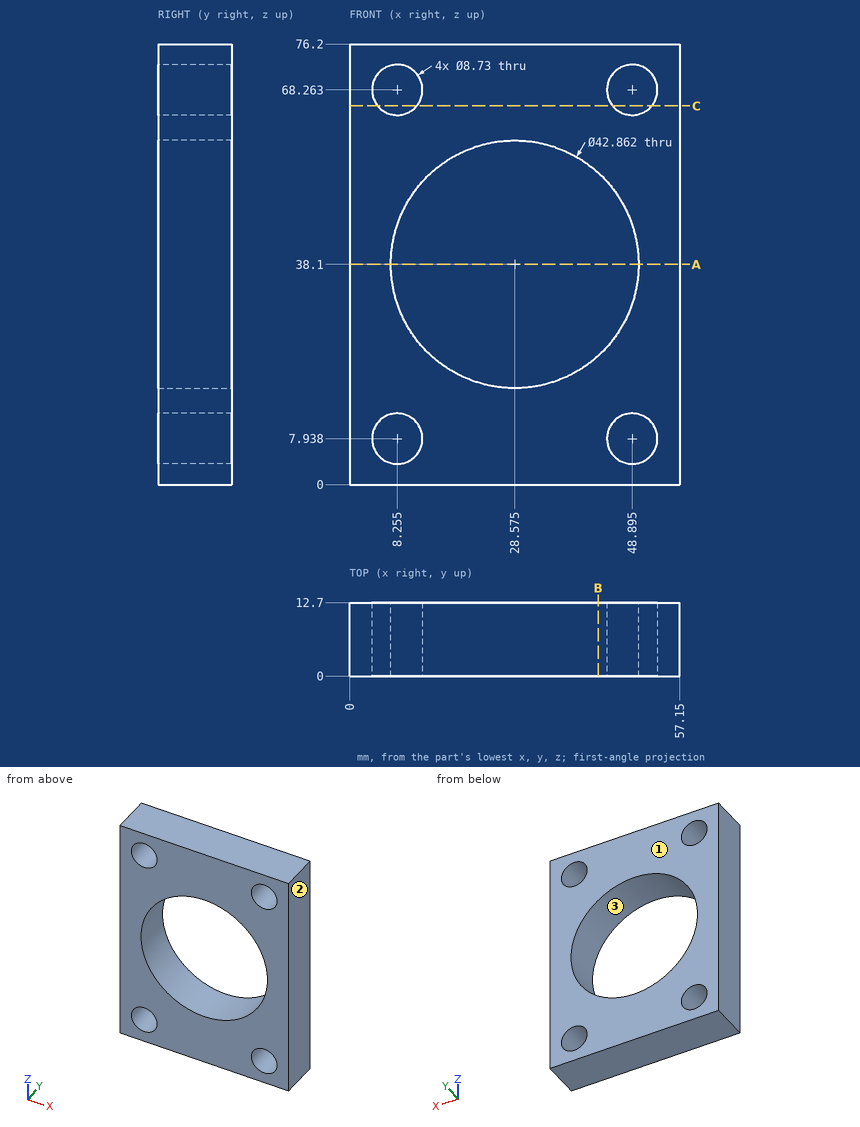
Geometry: see drawing. Coordinates: mm, zero at the bounding-box minimum. Give positions to 0.01 mm unless a question says otherwise; leave off trailing zeros. Write each loop counter-clockwise with the first axis right and the second up, starting at its lowest first coordinate (ties: lowest second). Pieces come first, ordered by that corner, then holes. Notation, with made-up numbers: (56.25, 28.25) -> (63.25, 28.25) arc R28 ccw to (63.25, 52.25) -> close; hole circle Ø1 at (1.25, 88.5). An arc over 180 degrees is marked (long way). Use one line per item in the form item = value. Start each with the question number.
1) Section query C-C on z = 65.5. Count the separate pieces of the cut face and the enclosed holes in it, then the cut area to 3 significant figures.
2) Section query A-A on z = 38.1. Return the cut outline in (x, y).
3) Section query B-B on x = 43. Return the cut outline in (y, z), then the cut area to 3 significant figures.
4) Draft query along X for the marked faces 1, 2 and 3. Return one class per face: pulls with the +X half, pulls with the -X half, needs draft (parallel to the pull), parting line crosses it, or undercut.
5) Ray query, probe 1 along X at (y, z) = (9.75, 68.5); probe 2 along Z at (x, y) = (11, 10.25) (1 decimal); probe 3 along Z at (x, y) = (7, 2.5). Return the intervals inside material, ascending. Write a range as from..to.
Outcome:
q1.separate_pieces = 3
q1.enclosed_holes = 0
q1.area = 554 mm^2
q2.outline = (0, 0) -> (7.14, 0) -> (7.14, 12.7) -> (0, 12.7) -> close; (50.01, 0) -> (57.15, 0) -> (57.15, 12.7) -> (50.01, 12.7) -> close
q3.outline = (0, 0) -> (12.7, 0) -> (12.7, 22.25) -> (0, 22.25) -> close; (0, 53.95) -> (12.7, 53.95) -> (12.7, 76.2) -> (0, 76.2) -> close
q3.area = 565 mm^2
q4.face_1 = needs draft
q4.face_2 = pulls with the +X half
q4.face_3 = undercut
q5.probe_1 = 0..3.9, 12.61..44.54, 53.25..57.15
q5.probe_2 = 0..4.5, 11.3..25.8, 50.4..64.9, 71.7..76.2
q5.probe_3 = 0..3.76, 12.12..64.08, 72.44..76.2
